from build123d import *

# Parameters (mm, degrees)
SKETCH1_R           = 16
BOSS_EXTRUDE1_DEPTH = 4.7
CUT_EXTRUDE1_DEPTH  = 1.7


with BuildPart() as part:
    # Sketch1 → Boss-Extrude1 (new body)
    with BuildSketch(Plane.XY):
        with BuildLine():
            Line((0, 0), (0, 75))
            add(Edge.make_bspline(
                [(0, 75), (-70, 75), (-70, 0)],
                knots=[0, 0, 0, 1, 1, 1], degree=2))
            Line((-70, 0), (0, 0))
        make_face()
        with Locations((-20, 49.85)):
            Circle(SKETCH1_R, mode=Mode.SUBTRACT)
    extrude(amount=BOSS_EXTRUDE1_DEPTH)

    # Sketch1_5 → Cut-Extrude1 (cut)
    with BuildSketch(Plane.XY):
        with BuildLine():
            Line((-18.197224362, 13), (-3.9, 13))
            Line((-3.9, 13), (-3.9, 7))
            Line((-3.9, 7), (-18.197224362, 7))
            ThreePointArc((-18.197224362, 7), (-20, 6.5), (-21.802775638, 7))
            Line((-21.802775638, 7), (-36.1, 7))
            Line((-36.1, 7), (-36.1, 13))
            Line((-36.1, 13), (-21.802775638, 13))
            ThreePointArc((-21.802775638, 13), (-20, 13.5), (-18.197224362, 13))
        make_face()
    extrude(amount=CUT_EXTRUDE1_DEPTH, mode=Mode.SUBTRACT)


solid = part.part
The model under review builds one solid part; all positions refer to its coordinate system, in mm. A direction names the side the tool comes from. Coordinates: 2 decimals unless noted, no trailing zeros. Answer in a Markdown table with one row per item.
(1) Insertion check: pin 1 (1.4 mm diameter, centred on x = -32, z = 0.5, fed in from +Y); pin 2 (2 mm diameter, centred on x = -22.5, y = 8.5, fed in from -Z); pin 3 (19 mm diameter, centred on x = -20, y = 49.85, fed in from -Z); pin 4 (1.4 mm diameter, centred on y = 8.5, z = 0.5, fed in from -X). Each pin has a flat end and moves straight along its axis. Give the tip position at first contact, or say it passes through.
Answers:
| item | result |
|---|---|
| pin 1 | y = 70.07 |
| pin 2 | z = 1.7 |
| pin 3 | through |
| pin 4 | x = -69.8 |
(2) The part is to be moulded in two halves that separate along X. For faces 3 (the flat face through (-35, 0, 2)), 4 (the flat face through (-36.1, 10, 1)), 5 (the cylindrical face through (-11.4, 63.34, 2.32)), 6 (the flat face through (0, 37, 2)), say which applies: +X half, -X half, draft (parallel to the pull), parting line (faces both ways), or undercut.
Answers:
| item | result |
|---|---|
| face 3 | draft |
| face 4 | undercut |
| face 5 | undercut |
| face 6 | +X half |
(3) Machinability: for faces 1 (the flat face through (-11, 7, 1)), 2 (the flat face through (-35, 30, 0)), which of the approach directions +Z, -Z, +X, -X, +Y, -Y give a long, thin tool a straight path to every point of the face, cutting with its end or side? Answer none if there is none.
Answers:
| item | result |
|---|---|
| face 1 | -Z |
| face 2 | -Z, +X, -X, +Y, -Y |
(4) Consider section A-A (z = 0.9). State how many separate pieces and enclosed holes the cut face has, plus the area to 3 significant figures.
Answers:
| item | result |
|---|---|
| separate pieces | 1 |
| enclosed holes | 2 |
| area | 3,380 mm² |
(5) Wall thickness on line 1 along Y through (x, z) = (-20, 0.35); line 2 along Y through (x, z) = (-30, 0.85); line 3 along X through (y, z) = (54.5, 4.25): over which ranges is each line inside the solid? List them lowest first.
Answers:
| item | result |
|---|---|
| line 1 | 0 to 6.5, 13.5 to 33.85, 65.85 to 73.2 |
| line 2 | 0 to 7, 13 to 37.36, 62.34 to 70.53 |
| line 3 | -54.06 to -35.31, -4.69 to 0 |
